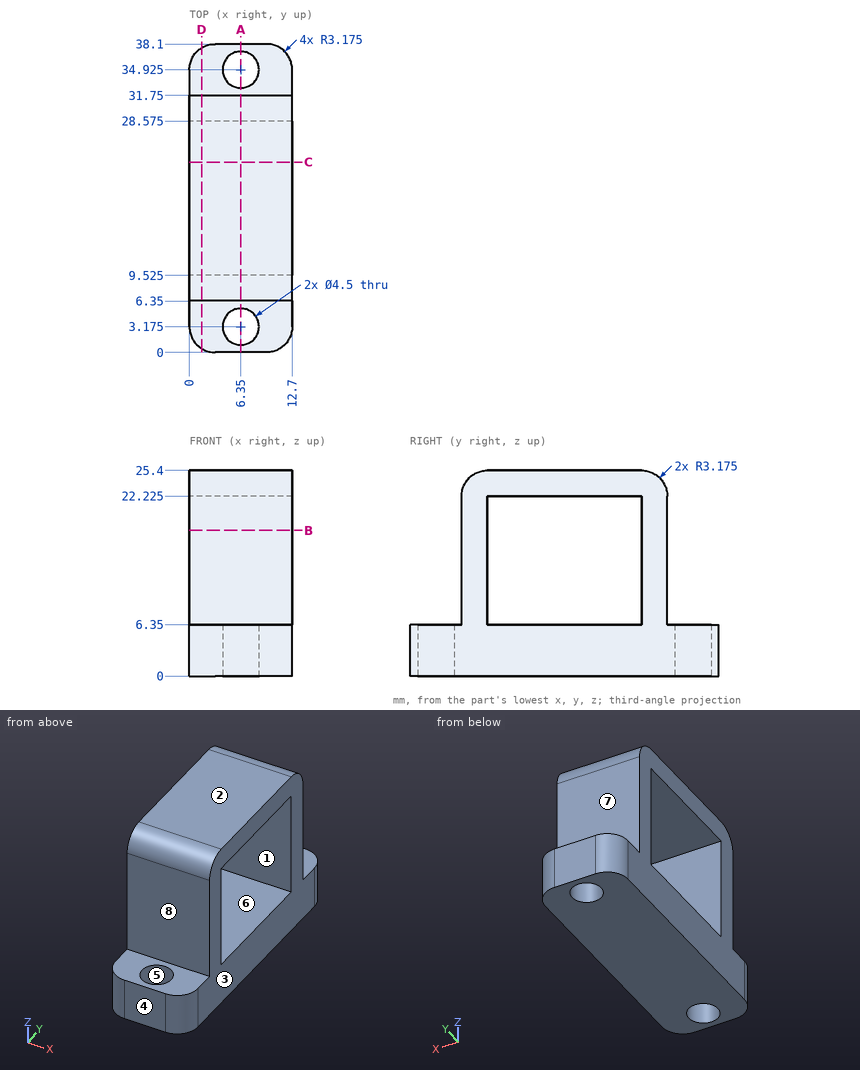
The figure shows three views and two pictorial views of one solid part (mm, origin at its lowest corner). Answer the questions. A direction names the side the tool comes from. Coordinates: 2 decimals unless noted, no trailing zeros. Loops run counter-clockwise (first coordinate to the right, second up) from the corner with the lowest first, then second, coordinate; pieces in that order, holes last. Notation, with made-up numbers: (-13, -37) -> (23, -37) arc R14 ccw to (23, -16) -> close; hole circle Ø5 at (-21.75, -31.5). An arc over 180 degrees is marked (long way). Use one line per item in the form item = value. Start each with the question number.
Item 1: Flat-ended cylindrical pins translate along their axes: pin 1 Ø1.9 at (x, y) = (3.5, 36) entering from +Z; pin 2 Ø5 at (x, z) = (9.5, 4.5) entering from -Y; pin 3 Ø1.5 at (x, y) = (7.5, 7.5) entering from +Z; pin 4 Ø4 at (x, z) = (6.5, 10.5) entering from -Y. Find the tip coordinate at first contact, or state that the pin passes through.
Item 2: The part is cut by section A-A on x = 6.35. Determine the outline of the cut face in (y, z) (3 decimals), then the cut area to 3 significant figures.
Item 3: Consider L1, parallel to Y at x = 6.35, z = 2.75 (3 decimals); L2, parallel to Z at x = 9.75, y = 24 (3 decimals); L3, parallel to Y at x = 7.5, z = 16 (3 decimals). Determine where each line is inside the solid, lowest interval first. Write a range as [from, to].
Item 4: The mould has two halves that part along Z. Classify the marked faces 1, 2 and 3: released by +Z, released by -Z, zero draft, split by the parting line, or undercut.
Item 5: The part is cut by section D-D on x = 1.5. Determine the outline of the cut face in (y, z) (3 decimals), then the cut area to 3 significant figures.
Item 6: The part is cut by section C-C on y = 23.5. Determine the outline of the cut face in (x, z) (3 decimals), then the cut area to 3 significant figures.
Item 7: A tool of negligible diameter and unlimited length cuts with its end or side. For the marked faces 4, 5, 6, 7 and 8, from which of +Z, -Z, +X, -X, +Y, -Y can it reach the whole face along a straight path? Write none if from no direction.
Item 8: The part is cut by section B-B on z = 18. Determine the outline of the cut face in (x, y) (3 decimals).
Answer key:
q1.pin_1 = 6.35
q1.pin_2 = 0
q1.pin_3 = 25.13
q1.pin_4 = 6.35
q2.outline = (0, 0) -> (0.925, 0) -> (0.925, 6.35) -> (0, 6.35) -> close; (5.425, 0) -> (32.675, 0) -> (32.675, 6.35) -> (31.75, 6.35) -> (31.75, 22.225) arc R3.175 ccw to (28.575, 25.4) -> (9.525, 25.4) arc R3.175 ccw to (6.35, 22.225) -> (6.35, 6.35) -> (5.425, 6.35) -> close; (37.175, 0) -> (38.1, 0) -> (38.1, 6.35) -> (37.175, 6.35) -> close; hole (9.525, 6.35) -> (28.575, 6.35) -> (28.575, 22.225) -> (9.525, 22.225) -> close
q2.area = 362 mm2
q3.L1 = [0, 0.925], [5.425, 32.675], [37.175, 38.1]
q3.L2 = [0, 6.35], [22.225, 25.4]
q3.L3 = [6.35, 9.525], [28.575, 31.75]
q4.face_1 = undercut
q4.face_2 = released by +Z
q4.face_3 = zero draft
q5.outline = (0.478, 0) -> (37.622, 0) -> (37.622, 6.35) -> (31.75, 6.35) -> (31.75, 22.225) arc R3.175 ccw to (28.575, 25.4) -> (9.525, 25.4) arc R3.175 ccw to (6.35, 22.225) -> (6.35, 6.35) -> (0.478, 6.35) -> close; hole (9.525, 6.35) -> (28.575, 6.35) -> (28.575, 22.225) -> (9.525, 22.225) -> close
q5.area = 413 mm2
q6.outline = (0, 0) -> (12.7, 0) -> (12.7, 6.35) -> (0, 6.35) -> close; (0, 22.225) -> (12.7, 22.225) -> (12.7, 25.4) -> (0, 25.4) -> close
q6.area = 121 mm2
q7.face_4 = +Z, -Z, +X, -X, -Y
q7.face_5 = +Z, -Z
q7.face_6 = +X, -X
q7.face_7 = +Z, +X, -X, +Y
q7.face_8 = +Z, +X, -X, -Y
q8.outline = (0, 6.35) -> (12.7, 6.35) -> (12.7, 9.525) -> (0, 9.525) -> close; (0, 28.575) -> (12.7, 28.575) -> (12.7, 31.75) -> (0, 31.75) -> close
